For this review, take the finished solid that the model builds, in its own axes (mm). A direction names the side the tool comes from. Round coordinates to 2 decimals unless told otherwise and drop trailing zeros. Write each loop counter-clockwise with the first axis right and the second up, starting at its lowest first coordinate (ties: lowest second). Pieces come first, ordered by that corner, then holes. Notation, with made-up numbers: (15, 71) -> (38, 71) arc R21 ccw to (38, 78) -> close; hole circle Ø11 at (-15.75, 77). An arc over 180 degrees is marked (long way). Write each question's results on one line, items separated by ' | '. Start each with the question number.
Item 1: Add section B-B (z = 0). State the section outline as (x, y) points, plus the area to 3 significant figures.
Item 2: Add section C-C (y = 1.5). State the section outline as (x, z) points.
Item 3: Tool access review of faces 4 (the flat face through (0, 2, -55)), 5 (the flat face through (0, 0, 0)), 6 (the cylindrical face through (-22.51, 2.46, 39.28)), 7 (the flat face through (11, 2, 55)): name each direction out of +Z, -Z, +X, -X, +Y, -Y from which nothing blocks a thin tool from reaching the whole face with its end or side.
Item 4: Add section A-A (x = 0). State the section outline as (y, z) points.
Item 5: To check wall thickness, follow line 1 along Z through (x, y) = (0, -2.6); line 2 along Z through (x, y) = (-20, -3.75); line 3 along Y through (x, z) = (5, -14). State the ranges of each line that lie inside material, in increasing order.
Item 6: Add section D-D (z = 20). State the section outline as (x, y) points, plus the area to 3 significant figures.
Item 7: Clearance check with flat-ended pins moving along their axes: pin 1 (1 mm diameter, centred on y = 1, z = -8.5, fed in from +X); pin 2 (1.5 mm diameter, centred on y = 1.5, z = -53.5, fed in from -X); pin 3 (8 mm diameter, centred on x = 0, z = -20, fed in from +Y). State where each tip first meets the part, or that it passes through.
Item 8: The part is to be moulded in two halves that separate along X. For faces 1 (the cylindrical face through (-17, -2, 0)), 2 (the flat face through (-36, 2, -35)), 3 (the flat face through (-40, 2, 0)), say which applies: +X half, -X half, draft (parallel to the pull), parting line (faces both ways), or undercut.
from build123d import *

# Parameters (mm, degrees)
F1_DEPTH = 5
F2_R     = 30
F3_DEPTH = 5
F4_R     = 3
F5_DEPTH = 5


with BuildPart() as f1:
    # F0 (on Front) → F1 (new body)
    with BuildSketch(Plane.XZ):
        Polygon((45, -60), (45, 0), (45, 60), (0, 60), (-45, 60), (-45, 0), (-45, -60), (0, -60), align=None)
    extrude(amount=F1_DEPTH)

    # F2 (on face) → F3 (join)
    with BuildSketch(Plane(origin=(0, 0, 0), x_dir=(-1, 0, 0), z_dir=(0, 1, 0))):
        with BuildLine():
            Line((-40, 55), (-40, -45))
            Line((-40, -45), (-18, -55))
            Line((-18, -55), (18, -55))
            Line((18, -55), (18, -50))
            ThreePointArc((18, -50), (22.393398, -39.393398), (33, -35))
            Line((33, -35), (40, -35))
            Line((40, -35), (40, 35))
            Line((40, 35), (33, 35))
            ThreePointArc((33, 35), (22.393398, 39.393398), (18, 50))
            Line((18, 50), (18, 55))
            Line((18, 55), (-40, 55))
        make_face()
        Circle(F2_R, mode=Mode.SUBTRACT)
    extrude(amount=F3_DEPTH)

    # F4 (on face) → F5 (cut)
    with BuildSketch(Plane(origin=(0, 0, 0), x_dir=(-1, 0, 0), z_dir=(0, 1, 0))):
        with Locations((-14.144271, -14.14)):
            Circle(F4_R)
        with Locations((-20, 0)):
            Circle(F4_R)
        with Locations((-14.144271, 14.14)):
            Circle(F4_R)
        with Locations((0, 20)):
            Circle(F4_R)
        with Locations((14.144271, 14.14)):
            Circle(F4_R)
        with Locations((20, 0)):
            Circle(F4_R)
        with Locations((14.144271, -14.14)):
            Circle(F4_R)
        with Locations((0, -20)):
            Circle(F4_R)
    extrude(amount=-F5_DEPTH, mode=Mode.SUBTRACT)


solid = f1.part
Responses:
1) outline: (-45, -5) -> (-23, -5) -> (-23, 0) -> (-30, 0) -> (-30, 5) -> (-40, 5) -> (-40, 0) -> (-45, 0) -> close; (-17, -5) -> (17, -5) -> (17, 0) -> (-17, 0) -> close; (23, -5) -> (45, -5) -> (45, 0) -> (40, 0) -> (40, 5) -> (30, 5) -> (30, 0) -> (23, 0) -> close | area: 490 mm^2
2) outline: (-40, -35) -> (-33, -35) arc R15 cw to (-18, -50) -> (-18, -55) -> (18, -55) -> (40, -45) -> (40, 55) -> (-18, 55) -> (-18, 50) arc R15 cw to (-33, 35) -> (-40, 35) -> close; hole circle Ø60 at (0, 0)
3) face 4: -Z, +X, -X, +Y | face 5: +Y | face 6: +Z, -X, +Y | face 7: +Z, +X, -X, +Y
4) outline: (-5, -60) -> (0, -60) -> (0, -55) -> (5, -55) -> (5, -30) -> (0, -30) -> (0, -23) -> (-5, -23) -> close; (-5, -17) -> (0, -17) -> (0, 17) -> (-5, 17) -> close; (-5, 23) -> (0, 23) -> (0, 30) -> (5, 30) -> (5, 55) -> (0, 55) -> (0, 60) -> (-5, 60) -> close
5) line 1: z = -60 to -23, -17 to 17, 23 to 60 | line 2: z = -60 to -3, 3 to 60 | line 3: y = -5 to 0
6) outline: (-45, -5) -> (-3, -5) -> (-3, 0) -> (-22.36, 0) -> (-22.36, 5) -> (-40, 5) -> (-40, 0) -> (-45, 0) -> close; (3, -5) -> (45, -5) -> (45, 0) -> (40, 0) -> (40, 5) -> (22.36, 5) -> (22.36, 0) -> (3, 0) -> close | area: 596 mm^2
7) pin 1: stops at x = 40 | pin 2: stops at x = -18 | pin 3: stops at y = 0
8) face 1: undercut | face 2: draft | face 3: -X half
